Autodesk Inventor part; units mm, degrees
ref_plane "YZ Plane" through (0, 0, 0) normal (1, 0, 0) x (0, 1, 0)
ref_plane "XZ Plane" through (0, 0, 0) normal (0, 1, 0) x (-1, 0, 0)
ref_plane "XY Plane" through (0, 0, 0) normal (0, 0, 1) x (1, 0, 0)
sketch "Sketch1" plane through (0, 0, 0) normal (0, 1, 0) x (-1, 0, 0)
  line L0 (-30, -30) -> (30, -30)
  line L1 (30, -30) -> (30, 30)
  line L2 (30, 30) -> (-30, 30)
  line L3 (-30, 30) -> (-30, -30)
  line L4 (-30, -30) -> (30, 30) construction
  line L5 (30, -30) -> (-30, 30) construction
  circle A0 centre (0, 0) radius 7.5
  dimension "d0" = 60
  dimension "d1" = 60
  dimension "d13" = 15
extrude "Extrusion1" add sketch "Sketch1" along normal blind 6
sketch "Sketch2" plane through (0, 6, 0) normal (0, 1, 0) x (1, 0, 0)
  line L0 (30, 30) -> (-30, 30)
  line L1 (-30, 30) -> (-30, -30)
  line L2 (-30, -30) -> (30, -30)
  line L3 (30, -30) -> (30, 30)
  line L4 (25, -25) -> (-25, -25)
  line L5 (-25, -25) -> (-25, 25)
  line L6 (-25, 25) -> (25, 25)
  line L7 (25, 25) -> (25, -25)
  line L8 (25, -25) -> (-25, 25) construction
  line L9 (-25, -25) -> (25, 25) construction
  line L10 (0, -25) -> (0, 25)
  line L11 (-25, 0) -> (25, 0)
  point P0 (0, 0)
  point P1 (0, 25)
  point P2 (-0.9499, 25.1888)
  dimension "d4" = 50
  dimension "d5" = 50
hole "Hole1" at (-25, 6, 0) at (25, 6, 0) direction (0, -1, 0) diameter 2.6 depth 10 tip angle 118
chamfer "Chamfer1" distance 2 angle 45 4 edges at (30, 3, 30) (30, 3, -30) (-30, 3, -30) (-30, 3, 30)
properties part number "00_XY_stage-CHUO_SEIKI_LD-647-R1-Top"
For this review, take the finished solid that the model builds, in its own axes (mm). Coordinates: 2 decimals unless noted, no trailing zeros. Loops run counter-clockwise (first coordinate to the right, second up) from the corner with the lowest first, then second, coordinate; pieces in that order, holes last.
1. Add section C-C, the plane y = 2.7. Give the boundary of the cut face in (x, z).
2. Add section D-D, the plane x = 25. Give the boundary of the cut face in (y, z).
3. For line 1 (X direction, y = 0.4, z = -1); line 2 (Z direction, x = 25, y = 2.9); line 3 (Z direction, x = -4.5, y = 2.35), list the stretches that pass through material, from the lowest coordinate up.
4. Mouldability with a two-part tool opening along Z and no side actions: class faces 1 (the flat face through (29, 3, 29)), 2 (the cylindrical face through (-23.73, 2.96, -0.28)), 3 (the flat face through (-29, 3, -29)) as +Z half, -Z half, draft (parallel to the pull), parting line (faces both ways), or undercut.
5. Add section A-A, the plane x = 0. Give the boundary of the cut face in (y, z), then the cut area to 3 significant figures.
6. Add section B-B, the plane z = 0. Give the boundary of the cut face in (x, y).
7. Insertion check: P1, Ø12, axis at x = 0, z = 0, coming from the -Y side; P2, Ø3, axis at x = 25, z = 0, coming from the -Y side. Each pin has a flat end and moves straight along its axis. Give the tip position at first contact, or say it passes through.
Result:
1. outline: (-30, -28) - (-28, -30) - (28, -30) - (30, -28) - (30, 28) - (28, 30) - (-28, 30) - (-30, 28) - close; hole circle Ø2.6 at (-25, 0); hole circle Ø15 at (0, 0); hole circle Ø2.6 at (25, 0)
2. outline: (0, -30) - (6, -30) - (6, -1.3) - (0, -1.3) - close; (0, 1.3) - (6, 1.3) - (6, 30) - (0, 30) - close
3. line 1: x = -30 to -25.83, -24.17 to -7.43, 7.43 to 24.17, 25.83 to 30
3. line 2: z = -30 to -1.3, 1.3 to 30
3. line 3: z = -30 to -6, 6 to 30
4. face 1: +Z half
4. face 2: undercut
4. face 3: -Z half
5. outline: (0, -30) - (6, -30) - (6, -7.5) - (0, -7.5) - close; (0, 7.5) - (6, 7.5) - (6, 30) - (0, 30) - close
5. area: 270 mm2
6. outline: (-30, 0) - (-26.3, 0) - (-26.3, 6) - (-30, 6) - close; (-23.7, 0) - (-7.5, 0) - (-7.5, 6) - (-23.7, 6) - close; (7.5, 0) - (23.7, 0) - (23.7, 6) - (7.5, 6) - close; (26.3, 0) - (30, 0) - (30, 6) - (26.3, 6) - close
7. P1: passes through
7. P2: stops at y = 0
